Job drawing, mm, ordinate dimensions from the low corner. One solid piece. A direction names the side the tool comes from. Give positions to 0.01 mm unless a question says otherwise; leave off trailing zeros. Write each loop counter-clockwise with the first axis right and the second up, starting at its lowest first coordinate (ties: lowest second). Pieces come first, ordered by that corner, then holes. Notation, with made-up numbers: M -37,38.25 L 0,38.25 A23 cw 0,64.25 Z; hole C -19,-34.75 d6. An arc over 180 degrees is marked long. Use a Markdown table: item, result.
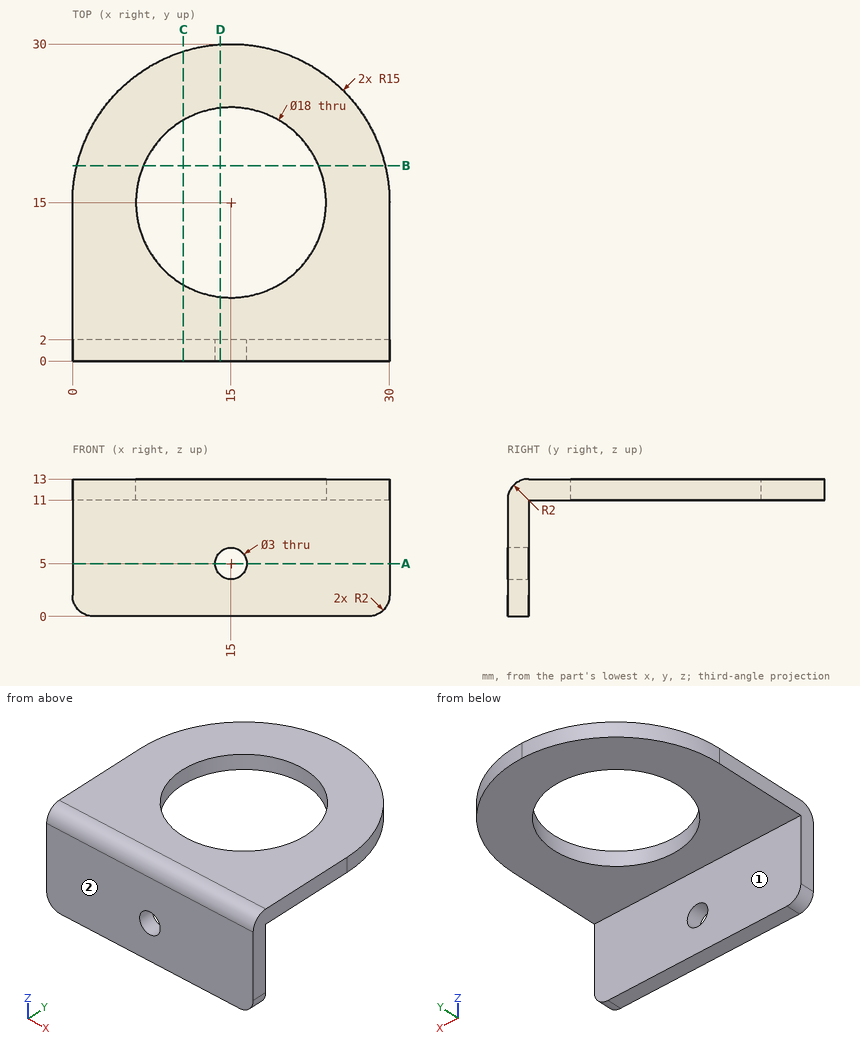
1. Drop flat-ended pins along their axis: P1, Ø4, axis at x = 19.5, z = 10, coming from the +Y side; P2, Ø1, axis at x = 18.5, z = 6, coming from the +Y side. Give the stop position or say it passes through.
Findings below:
| item | result |
|---|---|
| P1 | y = 29.74 |
| P2 | y = 2 |
2. Cut at D-D, the plane x = 14. Give the cut face in (y, z).
Findings below:
| item | result |
|---|---|
| outline | M 0,0 L 2,0 L 2,3.88 L 0,3.88 Z; M 0,6.12 L 2,6.12 L 2,11 L 6.06,11 L 6.06,13 L 2,13 A2 ccw 0,11 Z; M 23.94,11 L 29.97,11 L 29.97,13 L 23.94,13 Z |
3. Cut at A-A, the plane z = 5. Give the cut face in (x, y).
Findings below:
| item | result |
|---|---|
| outline | M 0,0 L 13.5,0 L 13.5,2 L 0,2 Z; M 16.5,0 L 30,0 L 30,2 L 16.5,2 Z |
4. Drill centre lines: L1, parallel to X at y = 0.55, z = 5; L2, parallel to Y at x = 26, z = 8.5; L3, parallel to Z at x = 2.5, y = 22. Where is each one in solid material? Low to high.
Findings below:
| item | result |
|---|---|
| L1 | 0 to 13.5, 16.5 to 30 |
| L2 | 0 to 2 |
| L3 | 11 to 13 |
5. Tool access for the marked faces 1 and 2: list every direction of +Z, -Z, +X, -X, +Y, -Y with a clear straight run to the whole face (end or side of a thin tool).
Findings below:
| item | result |
|---|---|
| face 1 | -Z, +X, -X, +Y |
| face 2 | +Z, -Z, +X, -X, -Y |
6. Cut at B-B, the plane y = 18.5. Give the cut face in (x, z).
Findings below:
| item | result |
|---|---|
| outline | M 0.41,11 L 6.71,11 L 6.71,13 L 0.41,13 Z; M 23.29,11 L 29.59,11 L 29.59,13 L 23.29,13 Z |
7. Cut at C-C, the plane x = 10.5. Give the cut face in (y, z).
Findings below:
| item | result |
|---|---|
| outline | M 0,0 L 2,0 L 2,11 L 7.21,11 L 7.21,13 L 2,13 A2 ccw 0,11 Z; M 22.79,11 L 29.31,11 L 29.31,13 L 22.79,13 Z |
